Work out the finished part from the listing and answer in its coordinate system (mm). A direction names the side the tool comes from. Give positions to 0.01 mm unless a question says otherwise; leave off trailing zeros. Order: outer loops, then holes, each group sorted by start corner. A loop starts at its lowest first (then second) coordinate and runs counter-clockwise, first axis right, second up. Notation, with made-up numbers: M -13,-32 L 15,-32 A15 ccw 15,-3 Z; hole C -20.75,59.25 d1. An arc over 180 degrees is marked long. One line per item, written item: value.
from build123d import *

# Parameters (mm, degrees)
EXTRUDE_1_DEPTH      = 12
CUT_EXTRUDE_2_DEPTH  = 7
SKETCH_4_W           = 12
SKETCH_4_H           = 56.291651246
EXTRUDE_2_DEPTH      = 85
EXTRUDE_3_DEPTH      = 12
CUT_EXTRUDE_4_DEPTH  = 12
FILLET_1_R           = 10
FILLET_2_R           = 10
SKETCH_8_R           = 2
CUT_EXTRUDE_9_DEPTH  = 5
CUT_EXTRUDE_7_DEPTH  = 7
SKETCH_3_R           = 2
CUT_EXTRUDE_8_DEPTH  = 5
EXTRUDE_START        = -12
EXTRUDE_5_DEPTH      = 12
SKETCH_13_R          = 3
CUT_EXTRUDE_11_DEPTH = 15


with BuildPart() as part:
    # 草图1 → 凸台-拉伸1 (new body)
    with BuildSketch(Plane(origin=(0, 0, 0), x_dir=(1, 0, 0), z_dir=(0, 1, 0))):
        with BuildLine():
            Line((16.25, -28.145825623), (0, 0))
            Line((0, 0), (16.25, 28.145825623))
            ThreePointArc((16.25, 28.145825623), (-32.5, 0), (16.25, -28.145825623))
        make_face()
        with BuildLine():
            Line((32.5, 0), (0, 0))
            Line((0, 0), (16.25, -28.145825623))
            ThreePointArc((16.25, -28.145825623), (28.145825623, -16.25), (32.5, 0))
        make_face()
        with BuildLine():
            Line((16.25, 28.145825623), (0, 0))
            Line((0, 0), (32.5, 0))
            ThreePointArc((32.5, 0), (28.145825623, 16.25), (16.25, 28.145825623))
        make_face()
        with BuildLine():
            ThreePointArc((16.25, 28.145825623), (28.145825623, 16.25), (32.5, 0))
            Line((32.5, 0), (50, 0))
            Line((50, 0), (50, 28.145825623))
            Line((50, 28.145825623), (16.25, 28.145825623))
        make_face()
        with BuildLine():
            Line((50, 0), (32.5, 0))
            ThreePointArc((32.5, 0), (28.145825623, -16.25), (16.25, -28.145825623))
            Line((16.25, -28.145825623), (50, -28.145825623))
            Line((50, -28.145825623), (50, 0))
        make_face()
    extrude(amount=EXTRUDE_1_DEPTH)

    # 草图2 → 切除-拉伸2 (cut)
    with BuildSketch(Plane(origin=(0, 12, 0), x_dir=(1, 0, 0), z_dir=(0, 1, 0))):
        Polygon((5, -8.660254038), (10, 0), (5, 8.660254038), (-5, 8.660254038), (-10, 0), (-5, -8.660254038), align=None)
    extrude(amount=-CUT_EXTRUDE_2_DEPTH, mode=Mode.SUBTRACT)

    # 草图4 → 凸台-拉伸2 (add)
    with BuildSketch(Plane.XZ):
        with Locations((44, 0)):
            Rectangle(SKETCH_4_W, SKETCH_4_H)
    extrude(amount=EXTRUDE_2_DEPTH)

    # 草图6 → 凸台-拉伸3 (add)
    with BuildSketch(Plane(origin=(50, 0, 0), x_dir=(0, 0, -1), z_dir=(1, 0, 0))):
        with BuildLine():
            ThreePointArc((-28.145825623, -21.75), (-32.5, -38), (-28.145825623, -54.25))
            Line((-28.145825623, -54.25), (-28.145825623, -21.75))
        make_face()
        with BuildLine():
            ThreePointArc((28.145825623, -54.25), (31.392589354, -46.411618966), (32.5, -38))
            ThreePointArc((32.5, -38), (31.392589354, -29.588381034), (28.145825623, -21.75))
            Line((28.145825623, -21.75), (28.145825623, -54.25))
        make_face()
    extrude(amount=-EXTRUDE_3_DEPTH)

    # 草图7 → 切除-拉伸4 (cut)
    with BuildSketch(Plane(origin=(50, 0, 0), x_dir=(0, 0, -1), z_dir=(1, 0, 0))):
        with BuildLine():
            Line((28.145825623, -85), (28.145825623, -54.25))
            ThreePointArc((28.145825623, -54.25), (0, -70.5), (-28.145825623, -54.25))
            Line((-28.145825623, -54.25), (-28.145825623, -85))
            Line((-28.145825623, -85), (28.145825623, -85))
        make_face()
    extrude(amount=-CUT_EXTRUDE_4_DEPTH, mode=Mode.SUBTRACT)

    # 圆角1
    fillet_1_edges = [part.edges().sort_by_distance(p)[0] for p in [
        (38, 0, 0),
    ]]
    fillet(fillet_1_edges, radius=FILLET_1_R)

    # 圆角2
    fillet_2_edges = [part.edges().sort_by_distance(p)[0] for p in [
        (50, 12, 0),
    ]]
    fillet(fillet_2_edges, radius=FILLET_2_R)

    # 草图8 → 切除-拉伸9 (cut)
    with BuildSketch(Plane(origin=(50, 0, 0), x_dir=(0, 0, -1), z_dir=(1, 0, 0))):
        with Locations((0, -38)):
            Circle(SKETCH_8_R)
        with Locations((0, -43.773502692)):
            Circle(SKETCH_8_R)
        with Locations((5, -35.113248654)):
            Circle(SKETCH_8_R)
        with Locations((-5, -35.113248654)):
            Circle(SKETCH_8_R)
    extrude(amount=-CUT_EXTRUDE_9_DEPTH, mode=Mode.SUBTRACT)

    # 草图10 → 切除-拉伸7 (cut)
    with BuildSketch(Plane.ZY.offset(-38)):
        Polygon((10, -38), (5, -29.339745962), (-5, -29.339745962), (-10, -38), (-5, -46.660254038), (5, -46.660254038), align=None)
    extrude(amount=-CUT_EXTRUDE_7_DEPTH, mode=Mode.SUBTRACT)

    # 草图3 → 切除-拉伸8 (cut)
    with BuildSketch(Plane.XZ):
        with Locations(Location((0, 0, 0), (0, 0, 270))):
            Circle(SKETCH_3_R)
        with Locations(Location((0, -5.773502692, 0), (0, 0, 270))):
            Circle(SKETCH_3_R)
        with Locations(Location((5, 2.886751346, 0), (0, 0, 270))):
            Circle(SKETCH_3_R)
        with Locations(Location((-5, 2.886751346, 0), (0, 0, 270))):
            Circle(SKETCH_3_R)
    extrude(amount=-CUT_EXTRUDE_8_DEPTH, mode=Mode.SUBTRACT)

    # 草图12 → 凸台-拉伸5 (add)
    with BuildSketch(Plane(origin=(0, 12, 0), x_dir=(1, 0, 0), z_dir=(0, 1, 0)).offset(EXTRUDE_START)):
        with BuildLine():
            ThreePointArc((-16.25, -28.145825623), (-28.145825623, -16.25), (-32.5, 0))
            Line((-32.5, 0), (-38, 0))
            Line((-38, 0), (-38, -28.145825623))
            Line((-38, -28.145825623), (-16.25, -28.145825623))
        make_face()
        with BuildLine():
            Line((-38, 0), (-32.5, 0))
            ThreePointArc((-32.5, 0), (-28.145825623, 16.25), (-16.25, 28.145825623))
            Line((-16.25, 28.145825623), (-38, 28.145825623))
            Line((-38, 28.145825623), (-38, 0))
        make_face()
    extrude(amount=EXTRUDE_5_DEPTH)

    # 草图13 → 切除-拉伸11 (cut)
    with BuildSketch(Plane.ZY.offset(38)):
        with Locations((-20, 6)):
            Circle(SKETCH_13_R)
        with Locations((20, 6)):
            Circle(SKETCH_13_R)
        with Locations((0, 6)):
            Circle(SKETCH_13_R)
    extrude(amount=-CUT_EXTRUDE_11_DEPTH, mode=Mode.SUBTRACT)


solid = part.part
(1) Determine the mould class of faces 1 (the cylindrical face through (-30.6, 4.2, 17.6)), 2 (the flat face through (0, 9, -8.66)), 3 (the cylindrical face through (35.15, -3.01, 0.39)), 4 (the flat face through (2, 5, -2)) for opening direction Y: pulls with the +Y half, pulls with the -Y half, needs draft (parallel to the pull), parting line crosses it, or undercut.
Findings:
face 1: undercut
face 2: needs draft
face 3: pulls with the -Y half
face 4: pulls with the +Y half
(2) Section D-D, the plane y = -15.5 is taken. Give the vertices of the cut face in (x, z).
Findings:
outline: M 38,-28.15 L 50,-28.15 L 50,28.15 L 38,28.15 Z
(3) Which of the six approach directions +Z, -Z, +X, -X, +Y, -Y give full straight-line access (tool end or side, diameter ignored) to faces 5 (the flat face through (37, -1, 28.146)), 6 (the flat face through (0, 9, 8.66)), 7 (the flat face through (-27, 6, -28.146)), 8 (the cylindrical face through (-30.6, 4.2, -22.4))?
Findings:
face 5: +Z, +X, +Y
face 6: +Y
face 7: -Z, -X, +Y, -Y
face 8: -X
(4) Given P1, Ø12, axis at x = -26.5, z = -19, coming from the -Y side; P2, Ø8.5, axis at x = -4.5, z = -2.5, coming from the +Y side; P3, Ø5, axis at y = -34, z = 4, coming from the -X side; P4, Ø12, axis at y = -44.5, z = -9.5, coming from the -X side, each flat-ended and moving along its own axis, determine where each tip first touches the part or whether it passes through.
Findings:
P1: stops at y = 0
P2: stops at y = 12
P3: stops at x = 45
P4: stops at x = 38
(5) Find the intervals of material crossed by probe 1 along Y at (x, z) = (-26.5, 0); probe 2 along X at (y, z) = (-21, -26); probe 3 along Y at (x, z) = (17, 25.5), in increasing order. Write a range as from..to.
Findings:
probe 1: y = 0..3, 9..12
probe 2: x = 38..50
probe 3: y = 0..12
(6) Section B-B, the plane x = 42.5 is taken. Give the vertices of the cut face in (y, z), then the cut area to 3 significant figures.
Findings:
outline: M -21.75,-28.15 L 11.68,-28.15 L 11.68,28.15 L -21.75,28.15 A32.5 ccw long Z; hole M -46.66,-5 L -38,-10 L -29.34,-5 L -29.34,5 L -38,10 L -46.66,5 Z
area: 4,290 mm^2
(7) Section A-A, the plane x = 0 is taken. Give the vertices of the cut face in (y, z), then the cut area to 3 significant figures.
Findings:
outline: M 0,-32.5 L 12,-32.5 L 12,-8.66 L 5,-8.66 L 5,-7.77 L 0,-7.77 Z; M 0,-3.77 L 5,-3.77 L 5,-2 L 0,-2 Z; M 0,2 L 5,2 L 5,8.66 L 12,8.66 L 12,32.5 L 0,32.5 Z
area: 619 mm^2
(8) Section C-C, the plane z = -12.5 is taken. Give the vertices of the cut face in (x, y), then the cut area to 3 significant figures.
Findings:
outline: M -38,0 L 28,0 A10 cw 38,-10 L 38,-68 L 50,-68 L 50,2 A10 ccw 40,12 L -38,12 Z
area: 1,870 mm^2
